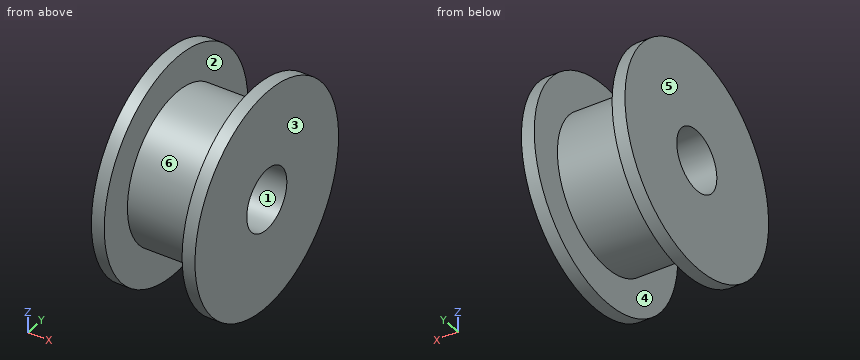
Autodesk Fusion 360 part; units mm, degrees
sketch "Sketch1" plane through (0, 0, 0) normal (0, 1, 0) x (1, 0, 0)
  line L0 (0, 0) -> (0, -5) construction
  line L1 (0, -2.5) -> (4.225, -2.5)
  line L2 (4.225, -2.5) -> (4.225, -8.96)
  line L3 (4.225, -8.96) -> (3.175, -8.96)
  line L4 (3.175, -8.96) -> (3.175, -6.07)
  line L5 (3.175, -6.07) -> (0, -6.07)
  line L6 (-4.225, -8.96) -> (-3.175, -8.96)
  line L7 (-3.175, -8.96) -> (-3.175, -6.07)
  line L8 (-3.175, -6.07) -> (0, -6.07)
  line L9 (0, -2.5) -> (-4.225, -2.5)
  line L10 (-4.225, -2.5) -> (-4.225, -8.96)
  dimension "d1" = 4.225
  dimension "d2" = 1.05
  dimension "d3" = 2.5
  dimension "d4" = 6.07
  dimension "d5" = 8.96
revolve "Revolve1" add sketch "Sketch1" angle 360 about axis through (1.75, 0, 0) along (1, 0, 0)
ref_plane "WorkPlane1" through (0, 0, 0) normal (-1, 0, 0) x (0, 0, 1)
sketch "Sketch2" plane through (0, 0, 0) normal (-1, 0, 0) x (0, 1, 0)
equation "d1 = ( 8.45 / 2 ) * 1 mm"
equation "d5 = ( 17.92 / 2 ) * 1 mm"
Source: CAD feature listing. Evaluate the final solid. Frame: model axes, mm. Face numbers are marked on the shaded views. A direction names the side the tool comes from. Coordinates: 2 decimals unless noted, no trailing zeros. Write each loop counter-clockwise with the first axis right and the second up, starting at its lowest first coordinate (ties: lowest second). Pieces come first, ordered by that corner, then holes. Notation, with made-up numbers: (55.5, -4) - (65.5, -4) arc R19 ccw to (65.5, 1) - close; hole circle Ø7 at (-36, 18.5). An arc over 180 degrees is marked (long way). Answer as a JSON object with one key per item and string values.
Q1. Draft query along X for the marked faces 3, 4, 5 and 6. Return one class per face: released by +X, released by -X, zero draft, split by the parting line, or undercut.
Ans:
{"face 3": "released by +X", "face 4": "undercut", "face 5": "released by -X", "face 6": "undercut"}
Q2. First-contact query: pin 1 Ø4 at (x, y) = (1.5, -1.5) entering from +Z; pin 2 Ø3 at (x, y) = (-1.5, 5) entering from -Z; pin 3 Ø1 at (x, y) = (1, -4.5) entering from -Z. Flat tips, straight axial feed; report the tip coordinate or a pass-through.
Ans:
{"pin 1": "stops at z = 8.95", "pin 2": "stops at z = -4.96", "pin 3": "stops at z = -4.57"}
Q3. Set-up query: the marked faces 1 and 2. Return all of +Z, -Z, +X, -X, +Y, -Y with unobstructed straight access to the full face (end or side cutting, diameter ignored); none if empty.
Ans:
{"face 1": "+X, -X", "face 2": "none"}
Q4. Section query D-D, the plane z = 6.5. Output: boundary loops of the cut face in (x, y) (3 decimals).
Ans:
{"outline": "(-4.225, -6.167) - (-3.175, -6.167) - (-3.175, 6.167) - (-4.225, 6.167) - close; (3.175, -6.167) - (4.225, -6.167) - (4.225, 6.167) - (3.175, 6.167) - close"}
Q5. Section query C-C, the plane x = -3.5. Output: boundary loops of the cut face in (y, z), plus the area to 3 significant figures.
Ans:
{"outline": "circle Ø17.92 at (0, 0); hole circle Ø5 at (0, 0)", "area": "233 mm2"}
Q6. Material intervals for line 1 (Y direction, x = -0.5, z = 0); line 2 (X direction, y = -1, z = -6.25) (3 decimals), sorted ascending. Write a range as [from, to].
Ans:
{"line 1": "y = [-6.07, -2.5], [2.5, 6.07]", "line 2": "x = [-4.225, -3.175], [3.175, 4.225]"}
Q7. Section query A-A, the plane y = 0. Output: boundary loops of the cut face in (x, z) (3 decimals), plus the area to 3 significant figures.
Ans:
{"outline": "(-4.225, -8.96) - (-3.175, -8.96) - (-3.175, -6.07) - (3.175, -6.07) - (3.175, -8.96) - (4.225, -8.96) - (4.225, -2.5) - (-4.225, -2.5) - close; (-4.225, 2.5) - (4.225, 2.5) - (4.225, 8.96) - (3.175, 8.96) - (3.175, 6.07) - (-3.175, 6.07) - (-3.175, 8.96) - (-4.225, 8.96) - close", "area": "72.5 mm2"}
